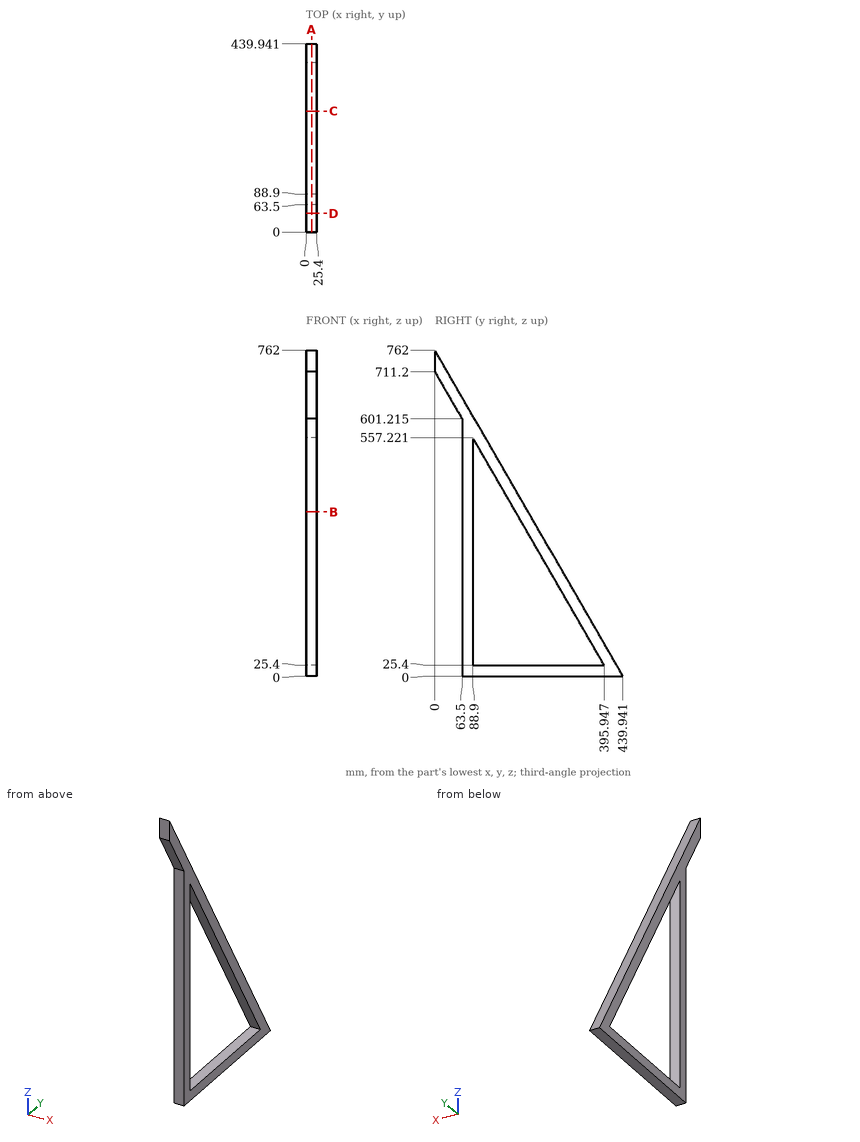
Answer from the drawing. Dimensions are ordinates in mm from the lowest x, y and z of the part. Coordinates: 2 decimals unless noted, no trailing zeros. Loops run counter-clockwise (first coordinate to the right, second up) from the corner with the lowest first, then second, coordinate; pieces in that order, holes last.
Q1. Consider probe 1 along Z at (x, y) = (1.5, 235); probe 2 along Y at (x, z) = (9.5, 75); probe 3 along Z at (x, y) = (24.25, 357). Determine where each line is inside the solid, lowest interval first.
Q2. The part is cut by section B-B on z = 383.5. Write down the section's boundary in (x, y), and give its area (3 significant figures).
Q3. The part is cut by section A-A on x = 13. Write down the section's boundary in (y, z) (1 decimal).
Q4. Each of these flat-tipped pins is pushed along its axis until it touches: pin 1 Ø10 at (x, y) = (8.5, 281) entering from +Z (1 decimal); pin 2 Ø8 at (x, z) = (20, 465) entering from +Y; pin 3 Ø12 at (x, z) = (6.5, 459.5) entering from -Y. Where does it stop, or does it pass through?
Q5. The part is cut by section D-D on y = 44. Write down the section's boundary in (x, z).
Q6. The part is cut by section C-C on y = 283. Write down the section's boundary in (x, z), and give its area (3 significant figures).
Results below:
1. probe 1: z = 0 to 25.4, 304.17 to 354.97
1. probe 2: y = 63.5 to 88.9, 367.31 to 396.64
1. probe 3: z = 0 to 25.4, 92.86 to 143.66
2. outline: (0, 63.5) - (25.4, 63.5) - (25.4, 88.9) - (0, 88.9) - close; (0, 189.2) - (25.4, 189.2) - (25.4, 218.53) - (0, 218.53) - close
2. area: 1,390 mm2
3. outline: (0, 711.2) - (63.5, 601.2) - (63.5, 0) - (439.9, 0) - (0, 762) - close; hole (88.9, 25.4) - (395.9, 25.4) - (88.9, 557.2) - close
4. pin 1: stops at z = 284
4. pin 2: stops at y = 173.78
4. pin 3: stops at y = 63.5
5. outline: (0, 634.99) - (25.4, 634.99) - (25.4, 685.79) - (0, 685.79) - close
6. outline: (0, 0) - (25.4, 0) - (25.4, 25.4) - (0, 25.4) - close; (0, 221.03) - (25.4, 221.03) - (25.4, 271.83) - (0, 271.83) - close
6. area: 1,940 mm2
